Check sheet for the modelled part. Datum: model origin and axes. Units: mm. A direction names the side the tool comes from. Coordinates: 2 decimals unless noted, no trailing zeros. Write each loop counter-clockwise with the first axis right and the second up, starting at its lowest first coordinate (ties: lowest second). Pieces come first, ordered by that corner, then holes. Notation, with made-up numbers: M 57,-13.75 L 96,-13.75 A19 cw 96,16.25 Z; hole C 54,75 d11. An arc over 180 degrees is marked long. Answer as CSV lines item,"result". Start each with the question number.
Q1. Sectioned sample at B-B, the plane x = 2016. Record the cut outline in (y, z).
Q2. Access from +Z, -Z, +X, -X, +Y, -Y to the whole of each face (thin tool, end or side, straight path). Record for faces 1 (the cylindrical face through (2177.804, -128.064, 31.875)), 2 (the cylindrical face through (2177.804, -127.002, 68.1)), 3 (the flat face through (2199, -122, 68.975)).
Q3. Thickness scan on line 1 along Z through (x, y) = (1626, -89); line 2 along Y through (x, z) = (1550, 51). Record the ranges inside material, lowest first. Write a range as from..to.
Q4. Depth check by flat-ended pin: pin 1 Ø8 at (y, z) = (-111.5, 35) entering from -X; pin 2 Ø2 at (x, y) = (2735, -94) entering from +Z; pin 3 Ø4 at (x, y) = (2075.5, -126.5) entering from -Z. Enter the tip coordinate at first touch or a pass-through.
Q5. Sectioned sample at C-C, the plane x = 2883.5. Record the cut outline in (y, z), then the cut area to 3 significant figures.
Q6. Sectioned sample at A-A, the plane z = 48.5. Record the cut outline in (x, y) (3 decimals).
from build123d import *

# Parameters (mm, degrees)
EXTRUDE_1_DEPTH     = 100
SKETCH_2_R          = 30
CUT_EXTRUDE_1_DEPTH = 100
SKETCH_3_R          = 32.5
SKETCH_3_R_2        = 30
EXTRUDE_2_DEPTH     = 5
EXTRUDE_START       = 5
SKETCH_4_R          = 32.5
SKETCH_4_R_2        = 30
EXTRUDE_3_DEPTH     = 5
SKETCH_5_R          = 30
CUT_EXTRUDE_2_DEPTH = 248
SKETCH_6_R          = 35
SKETCH_6_R_2        = 30
EXTRUDE_4_DEPTH     = 5
SKETCH_7_R          = 35
SKETCH_7_R_2        = 30
EXTRUDE_5_DEPTH     = 5
SCALE1_SCALE        = 0.345


with BuildPart() as part:
    # 草图1 → 凸台-拉伸1 (new body)
    with BuildSketch(Plane.XY):
        with BuildLine():
            Line((-60.1323511, -127.533248731), (739.8676489, -277.533248731))
            Line((739.8676489, -277.533248731), (4439.8676489, -277.533248731))
            ThreePointArc((4439.8676489, -277.533248731), (4514.8676489, -202.533248731), (4439.8676489, -127.533248731))
            Line((4439.8676489, -127.533248731), (3639.8676489, 22.466751269))
            Line((3639.8676489, 22.466751269), (-60.1323511, 22.466751269))
            ThreePointArc((-60.1323511, 22.466751269), (-135.1323511, -52.533248731), (-60.1323511, -127.533248731))
        make_face()
    extrude(amount=EXTRUDE_1_DEPTH)

    # 草图2 → 切除-拉伸1 (cut)
    with BuildSketch(Plane.XY.offset(100)):
        with Locations((-60.1323511, -52.533248731)):
            Circle(SKETCH_2_R)
        with Locations((4439.8676489, -202.533248731)):
            Circle(SKETCH_2_R)
    extrude(amount=-CUT_EXTRUDE_1_DEPTH, mode=Mode.SUBTRACT)

    # 草图3 → 凸台-拉伸2 (add)
    # profile 1 of 2: a face of its own
    with BuildSketch(Plane(origin=(0, 0, 0), x_dir=(-1, 0, 0), z_dir=(0, 0, -1))):
        with Locations(Location((-4439.8676489, -202.533248731, 0), (0, 0, 180))):
            Circle(SKETCH_3_R)
        with Locations(Location((-4439.8676489, -202.533248731, 0), (0, 0, 180))):
            Circle(SKETCH_3_R_2, mode=Mode.SUBTRACT)
    # profile 2 of 2: a face of its own
    with BuildSketch(Plane(origin=(0, 0, 0), x_dir=(-1, 0, 0), z_dir=(0, 0, -1))):
        with Locations(Location((60.1323511, -52.533248731, 0), (0, 0, 180))):
            Circle(SKETCH_3_R)
        with Locations(Location((60.1323511, -52.533248731, 0), (0, 0, 180))):
            Circle(SKETCH_3_R_2, mode=Mode.SUBTRACT)
    extrude(amount=EXTRUDE_2_DEPTH)

    # 草图4 → 凸台-拉伸3 (add)
    # profile 1 of 2: a face of its own
    with BuildSketch(Plane.XY.offset(100).offset(EXTRUDE_START)):
        with Locations((-60.1323511, -52.533248731)):
            Circle(SKETCH_4_R)
        with Locations((-60.1323511, -52.533248731)):
            Circle(SKETCH_4_R_2, mode=Mode.SUBTRACT)
    # profile 2 of 2: a face of its own
    with BuildSketch(Plane.XY.offset(100).offset(EXTRUDE_START)):
        with Locations((4439.8676489, -202.533248731)):
            Circle(SKETCH_4_R)
        with Locations((4439.8676489, -202.533248731)):
            Circle(SKETCH_4_R_2, mode=Mode.SUBTRACT)
    extrude(amount=-EXTRUDE_3_DEPTH)

    # 草图5 → 切除-拉伸2 (cut)
    with BuildSketch(Plane(origin=(0, 0, 0), x_dir=(-1, 0, 0), z_dir=(0, 0, -1))):
        with Locations((-2189.8676489, -127.533248731)):
            Circle(SKETCH_5_R)
    extrude(amount=-CUT_EXTRUDE_2_DEPTH, mode=Mode.SUBTRACT)

    # 草图6 → 凸台-拉伸4 (add)
    with BuildSketch(Plane(origin=(0, 0, 0), x_dir=(-1, 0, 0), z_dir=(0, 0, -1)).offset(EXTRUDE_START)):
        with Locations(Location((-2189.8676489, -127.533248731, 0), (0, 0, 180))):
            Circle(SKETCH_6_R)
        with Locations((-2189.8676489, -127.533248731)):
            Circle(SKETCH_6_R_2, mode=Mode.SUBTRACT)
    extrude(amount=-EXTRUDE_4_DEPTH)

    # 草图7 → 凸台-拉伸5 (add)
    with BuildSketch(Plane.XY.offset(100)):
        with Locations((2189.8676489, -127.533248731)):
            Circle(SKETCH_7_R)
        with Locations(Location((2189.8676489, -127.533248731, 0), (0, 0, 180))):
            Circle(SKETCH_7_R_2, mode=Mode.SUBTRACT)
    extrude(amount=EXTRUDE_5_DEPTH)


with BuildPart() as part_1:
    # Scale1: scaled about (2189.8676489, -127.533248731, 50)
    add(part.part.scale(SCALE1_SCALE).moved(Location((1434.36331003, -83.534277919, 32.75))))


solid = part_1.part
Output:
1,outline,"M -179.28,32.75 L -75.78,32.75 L -75.78,67.25 L -179.28,67.25 Z"
2,face 1,"-Z"
2,face 2,"+Z"
2,face 3,"+Z, +X, -X, +Y, -Y"
3,line 1,"z = 32.75..67.25"
3,line 2,"y = -153.1..-75.78"
4,pin 1,"stops at x = 1388.41"
4,pin 2,"stops at z = 67.25"
4,pin 3,"stops at z = 32.75"
5,outline,"M -179.28,32.75 L -112.04,32.75 L -112.04,67.25 L -179.28,67.25 Z"
5,area,"2,320 mm^2"
6,outline,"M 1413.618,-127.533 L 1689.618,-179.283 L 2966.118,-179.283 A25.875 ccw 2966.118,-127.533 L 2690.118,-75.783 L 1413.618,-75.783 A25.875 ccw Z; hole C 1413.618,-101.658 d20.7; hole C 2189.868,-127.533 d20.7; hole C 2966.118,-153.408 d20.7"
